Model file for the job. Use its own axes, mm. A direction names the side the tool comes from. Round coordinates to 2 decimals unless told otherwise and drop trailing zeros. Write each loop counter-clockwise with the first axis right and the second up, starting at its lowest first coordinate (ties: lowest second). Pieces come first, ordered by that corner, then holes. Notation, with made-up numbers: (42, -4) - (87, -4) arc R18 cw to (87, 25) - close; hole circle Ø7 at (74.5, 6.25). An arc over 180 degrees is marked (long way). Answer as a JSON object with one key per item and string values. Group by question number.
from build123d import *

# Parameters (mm, degrees)
F0_W     = 140
F0_H     = 77
F0_R     = 4
F0_W_2   = 45
F0_H_2   = 45
F0_R_2   = 2
F1_DEPTH = 3
F2_W     = 140
F2_H     = 77
F2_R     = 2
F3_DEPTH = 10
F4_W     = 140
F4_H     = 77
F4_W_2   = 136.839989
F4_H_2   = 74
F5_DEPTH = 1.5
F6_R     = 2
F7_SIZE  = 2


with BuildPart() as f1:
    # F0 (on Top) → F1 (new body)
    with BuildSketch(Plane.XY):
        Rectangle(F0_W, F0_H)
        with Locations((-62, 0)):
            Circle(F0_R, mode=Mode.SUBTRACT)
        Rectangle(F0_W_2, F0_H_2, mode=Mode.SUBTRACT)
        with Locations((62, 0)):
            Circle(F0_R, mode=Mode.SUBTRACT)
        with Locations((-62, 0)):
            Circle(F0_R)
        with Locations((-62, 0)):
            Circle(F0_R_2, mode=Mode.SUBTRACT)
        with Locations((62, 0)):
            Circle(F0_R)
        with Locations((62, 0)):
            Circle(F0_R_2, mode=Mode.SUBTRACT)
    extrude(amount=F1_DEPTH)

    # F2 (on face) → F3 (join)
    with BuildSketch(Plane(origin=(0, 0, 0), x_dir=(1, 0, 0), z_dir=(0, 0, -1))):
        Rectangle(F2_W, F2_H)
        Polygon((-67, 4), (-67, 35.5), (67, 35.5), (67, 4), (67, -4), (67, -35.5), (-67, -35.5), (-67, -4), align=None, mode=Mode.SUBTRACT)
        with BuildLine():
            ThreePointArc((-58, 0), (-59.171573, 2.828427), (-62, 4))
            ThreePointArc((-62, 4), (-66, 0), (-62, -4))
            ThreePointArc((-62, -4), (-59.171573, -2.828427), (-58, 0))
        make_face()
        with Locations((-62, 0)):
            Circle(F2_R, mode=Mode.SUBTRACT)
        with BuildLine():
            ThreePointArc((66, 0), (64.828427, 2.828427), (62, 4))
            ThreePointArc((62, 4), (58, 0), (62, -4))
            ThreePointArc((62, -4), (64.828427, -2.828427), (66, 0))
        make_face()
        with Locations((62, 0)):
            Circle(F2_R, mode=Mode.SUBTRACT)
        with BuildLine():
            Line((-62, 4), (-67, 4))
            Line((-67, 4), (-67, -4))
            Line((-67, -4), (-62, -4))
            ThreePointArc((-62, -4), (-66, 0), (-62, 4))
        make_face()
        with BuildLine():
            Line((67, -4), (67, 4))
            Line((67, 4), (62, 4))
            ThreePointArc((62, 4), (64.828427, 2.828427), (66, 0))
            ThreePointArc((66, 0), (64.828427, -2.828427), (62, -4))
            Line((62, -4), (67, -4))
        make_face()
    extrude(amount=F3_DEPTH)

    # F4 (on face) → F5 (join)
    with BuildSketch(Plane(origin=(0, 0, -10), x_dir=(1, 0, 0), z_dir=(0, 0, -1))):
        Rectangle(F4_W, F4_H)
        with Locations((-0.080005, 0)):
            Rectangle(F4_W_2, F4_H_2, mode=Mode.SUBTRACT)
    extrude(amount=F5_DEPTH)

    # F6
    f6_edges = [f1.edges().sort_by_distance(p)[0] for p in [
        (0, -38.5, 3),
        (70, 0, 3),
        (0, 38.5, 3),
        (-70, 0, 3),
        (-70, 38.5, -4.25),
        (-70, -38.5, -4.25),
        (70, -38.5, -4.25),
        (70, 38.5, -4.25),
    ]]
    fillet(f6_edges, radius=F6_R)

    # F7
    f7_edges = [f1.edges().sort_by_distance(p)[0] for p in [
        (-64, 0, 3),
        (60, 0, 3),
    ]]
    chamfer(f7_edges, length=F7_SIZE)


solid = f1.part
(1) Slice it at B-B (z = -7). Write the cut outline in (x, y).
(2) 3-axis set-ups, long thin cutter, end or side, ignore diameter. For faces 4 (the flat face through (-64, -4, -5)), 5 (the flat face through (0, 22.5, 1)), 6 (the flat face through (70, 1, -5)): which of +Z, -Z, +X, -X, +Y, -Y reach the whole face in a straight line?
(3) Flat gauge pins, fed straight in: pin 1 (21.5 mm diameter, centred on x = -9.5, y = 11.5, fed in from -Z); pin 2 (8 mm diameter, centred on x = 32.5, y = 8.5, fed in from -Z); pin 3 (5 mm diameter, centred on x = -62, y = 0, fed in from -Z). Where does each tip first touch, or does it go through?
(4) Drill centre lines: line 1 (X direction, y = 0, z = -4); line 2 (Y direction, x = 62, z = -1.25); line 3 (Y direction, x = -27, z = -3.5). Where is each one in solid material? Low to high. Write a range as from..to.
(5) Slice it at D-D (x = 47.5). Write the cut outline in (y, z), then the cut area to 3 significant figures.
(6) Slice it at C-C (x = -12.5). Write the cut outline in (y, z).
(7) Pull direction Y, two halves, no side cores. Call faces 1 (the flat face through (-70, 1, -5)), 2 (the flat face through (-1, -38.5, -5)), 3 (the flat face through (65, -4, -5)): pulls with the +Y half, pulls with the -Y half, needs draft (parallel to the pull), parting line crosses it, or undercut.
(8) Slice it at A-A (y = 20.5). Write the cut outline in (x, z), then the cut area to 3 significant figures.
Answer:
{
 "1": {"outline": "(-70, -36.5) arc R2 ccw to (-68, -38.5) - (68, -38.5) arc R2 ccw to (70, -36.5) - (70, 36.5) arc R2 ccw to (68, 38.5) - (-68, 38.5) arc R2 ccw to (-70, 36.5) - close; hole (-67, -35.5) - (67, -35.5) - (67, -4) - (62, -4) arc R4 cw to (62, 4) - (67, 4) - (67, 35.5) - (-67, 35.5) - (-67, 4) - (-62, 4) arc R4 cw to (-62, -4) - (-67, -4) - close; hole circle Ø4 at (-62, 0); hole circle Ø4 at (62, 0)"},
 "2": {"face 4": "-Z", "face 5": "+Z, -Z", "face 6": "+Z, -Z, +X, +Y, -Y"},
 "3": {"pin 1": "through", "pin 2": "z = 0", "pin 3": "z = -10"},
 "4": {"line 1": "-70..-64, -60..-58, 58..60, 64..70", "line 2": "-38.5..-35.5, -4..-2, 2..4, 35.5..38.5", "line 3": "-38.5..-35.5, 35.5..38.5"},
 "5": {"outline": "(-38.5, -11.5) - (-37, -11.5) - (-37, -10) - (-35.5, -10) - (-35.5, 0) - (35.5, 0) - (35.5, -10) - (37, -10) - (37, -11.5) - (38.5, -11.5) - (38.5, 1) arc R2 ccw to (36.5, 3) - (-36.5, 3) arc R2 ccw to (-38.5, 1) - close", "area": "294 mm²"},
 "6": {"outline": "(-38.5, -11.5) - (-37, -11.5) - (-37, -10) - (-35.5, -10) - (-35.5, 0) - (-22.5, 0) - (-22.5, 3) - (-36.5, 3) arc R2 ccw to (-38.5, 1) - close; (22.5, 0) - (35.5, 0) - (35.5, -10) - (37, -10) - (37, -11.5) - (38.5, -11.5) - (38.5, 1) arc R2 ccw to (36.5, 3) - (22.5, 3) - close"},
 "7": {"face 1": "needs draft", "face 2": "pulls with the -Y half", "face 3": "undercut"},
 "8": {"outline": "(-70, -11.5) - (-68.5, -11.5) - (-68.5, -10) - (-67, -10) - (-67, 0) - (-22.5, 0) - (-22.5, 3) - (-68, 3) arc R2 ccw to (-70, 1) - close; (22.5, 0) - (67, 0) - (67, -10) - (68.34, -10) - (68.34, -11.5) - (70, -11.5) - (70, 1) arc R2 ccw to (68, 3) - (22.5, 3) - close", "area": "348 mm²"}
}
